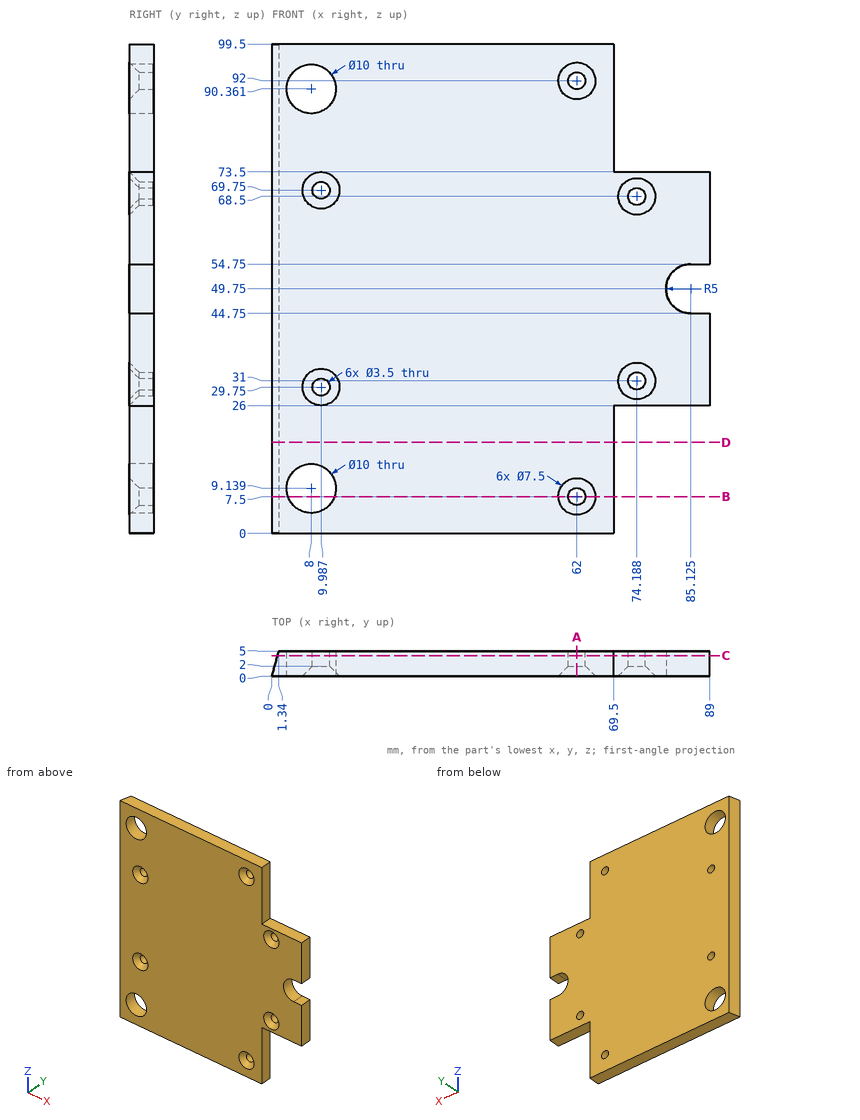
For this review, use the dimensioned drawing (mm, ordinates from the lowest corner) and the shaded views. Coordinates: 2 decimals unless noted, no trailing zeros. Loops run counter-clockwise (first coordinate to the right, second up) from the corner with the lowest first, then second, coordinate; pieces in that order, holes last. Notation, with made-up numbers: (-15.5, -31) -> (14.5, -31) arc R26 ccw to (14.5, -7) -> close; hole circle Ø3 at (49, 6.25). An arc over 180 degrees is marked (long way). Write each question's results on one line, items separated by ' | '.
Q1. To check wall thickness, follow line 1 along Z through (x, y) = (62, 4.35); line 2 along Z through (x, y) = (63, 1.5) (1 decimal); line 3 along Z through (x, y) = (11.5, 2.9) (1 decimal). State the ranges of each line that lie inside material, in increasing order. Write a range as [from, to].
Taken from the geometry:
line 1: [0, 5.75], [9.25, 90.25], [93.75, 99.5] | line 2: [0, 5.5], [9.5, 90], [94, 99.5] | line 3: [0, 5.6], [12.7, 28.9], [30.6, 68.9], [70.6, 86.8], [93.9, 99.5]
Q2. Add section C-C, the plane y = 4.15. Count the separate pieces of the cut face and the enclosed holes in it, then the cut area to 3 significant figures.
Taken from the geometry:
separate pieces: 1 | enclosed holes: 8 | area: 7,440 mm²
Q3. Add section D-D, the plane z = 18.5. State the section outline as (x, y) points, then the cut area to 3 significant figures.
Taken from the geometry:
outline: (0, 0) -> (69.5, 0) -> (69.5, 5) -> (1.34, 5) -> close | area: 344 mm²
Q4. For pin 1 Ø3 at (x, y) = (87.5, 3.5) entering from +Z; pin 2 Ø2.5 at (y, z) = (2, 85.5) entering from +X; pin 3 Ø4.5 at (x, z) = (9.99, 69.75) entering from -Y (1 decimal), all flat-tipped, find the tip position at first contact; note any pin that passes through.
Taken from the geometry:
pin 1: z = 73.5 | pin 2: x = 69.5 | pin 3: y = 1.5
Q5. Add section B-B, the plane z = 7.5. State the section outline as (x, y) points.
Taken from the geometry:
outline: (0, 0) -> (3.28, 0) -> (3.28, 5) -> (1.34, 5) -> close; (12.72, 0) -> (58.25, 0) -> (60.25, 2) -> (60.25, 5) -> (12.72, 5) -> close; (63.75, 2) -> (65.75, 0) -> (69.5, 0) -> (69.5, 5) -> (63.75, 5) -> close
Q6. Add section A-A, the plane x = 62. State the section outline as (y, z) points.
Taken from the geometry:
outline: (0, 0) -> (5, 0) -> (5, 5.75) -> (2, 5.75) -> (0, 3.75) -> close; (0, 11.25) -> (2, 9.25) -> (5, 9.25) -> (5, 90.25) -> (2, 90.25) -> (0, 88.25) -> close; (0, 95.75) -> (2, 93.75) -> (5, 93.75) -> (5, 99.5) -> (0, 99.5) -> close
